CAD build for the part. Positions are in the model's coordinates, mm. Round coordinates to 2 decimals unless told otherwise and drop trailing zeros. Order: outer loops, then holes, each group sorted by start corner. A loop starts at its lowest first (then second) coordinate and runs counter-clockwise, first axis right, second up. Notation, with made-up numbers: (41.5, -16.75) -> (74.5, -16.75) arc R24 ccw to (74.5, -0.75) -> close; hole circle Ø2 at (41, 67). An arc over 180 degrees is marked (long way). Answer as CSV lines item,"result". Start each with the question number.
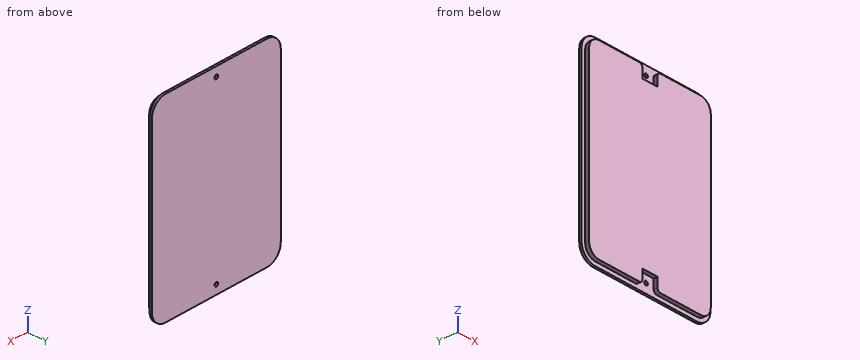
Autodesk Inventor part; units mm, degrees
ref_plane "YZ Plane" through (0, 0, 0) normal (1, 0, 0) x (0, 1, 0)
ref_plane "XZ Plane" through (0, 0, 0) normal (0, 1, 0) x (-1, 0, 0)
ref_plane "XY Plane" through (0, 0, 0) normal (0, 0, 1) x (1, 0, 0)
sketch "Sketch1" plane through (0, 0, 0) normal (0, 1, 0) x (-1, 0, 0)
  line L0 (0, 0) -> (178, 0)
  line L1 (178, 0) -> (178, -248)
  line L2 (178, -248) -> (0, -248)
  line L3 (0, -248) -> (0, 0)
  dimension "d0" = 178
  dimension "d1" = 248
extrude "Extrusion1" add sketch "Sketch1" along normal blind 3
fillet "Fillet1" radius 19 4 edges at (0, 1.5, 0) (-178, 1.5, 0) (0, 1.5, -248) (-178, 1.5, -248)
sketch "Sketch2" plane through (0, 0, 0) normal (0, -1, 0) x (1, 0, 0)
  arc A0 (-178, -229) -> (-159, -248) centre (-159, -229) ccw
  line L0 (-19, -248) -> (-159, -248)
  arc A1 (-19, -248) -> (0, -229) centre (-19, -229) ccw
  line L1 (0, -19) -> (0, -229)
  arc A2 (0, -19) -> (-19, 0) centre (-19, -19) ccw
  line L2 (-159, 0) -> (-19, 0)
  arc A3 (-159, 0) -> (-178, -19) centre (-159, -19) ccw
  line L3 (-178, -229) -> (-178, -19)
  arc A4 (-159, -5) -> (-173, -19) centre (-159, -19) ccw
  line L4 (-159, -5) -> (-19, -5)
  arc A5 (-5, -19) -> (-19, -5) centre (-19, -19) ccw
  line L5 (-5, -19) -> (-5, -229)
  arc A6 (-19, -243) -> (-5, -229) centre (-19, -229) ccw
  line L6 (-19, -243) -> (-159, -243)
  arc A7 (-173, -229) -> (-159, -243) centre (-159, -229) ccw
  line L7 (-173, -229) -> (-173, -19)
  line L8 (-78.5, -243) -> (-99.5, -243)
  line L9 (-99.5, -243) -> (-99.5, -227)
  line L10 (-99.5, -227) -> (-78.5, -227)
  line L11 (-78.5, -227) -> (-78.5, -243)
  line L12 (-173, -124) -> (-5, -124) construction
  line L13 (-78.5, -5) -> (-99.5, -5)
  line L14 (-99.5, -5) -> (-99.5, -21)
  line L15 (-99.5, -21) -> (-78.5, -21)
  line L16 (-78.5, -21) -> (-78.5, -5)
  circle A8 centre (-89, -11.5) radius 2.5
  line L17 (-89, -227) -> (-89, -21) construction
  circle A9 centre (-89, -236.5) radius 2.5
  point P0 (0, 0)
  point P1 (-89, -243)
  point P2 (-89, -5)
  point P3 (-99.5, -243)
  point P4 (-78.5, -5)
  point P5 (-99.5, -5)
  dimension "d12" = 21
  dimension "d13" = 21
  dimension "d14" = 5
  dimension "d16" = 5
  dimension "d18" = 225
extrude "Extrusion2" add sketch "Sketch2" along normal blind 5 contours L4 L14 L15 L16 A5 L5 A6 L6 L11 L10 L9 A7 L7 A4
extrude "Extrusion4" cut sketch "Sketch2" against normal up to surface (3 mm away) contours A8 | A9
fillet "Fillet2" radius 4 4 edges at (-99.5, -2.5, -243) (-78.5, -2.5, -243) (-99.5, -2.5, -5) (-78.5, -2.5, -5)
equation "\"d5\" = d16"
equation "\"d19\" = d16"
properties part number "case5_3DPrint"
Item 1: Band-saw the part on D-D, the plane z = -236.5. Give the cut face in (x, y).
Item 2: Band-saw the part on B-B, the plane y = -3.5. Give the cut face in (x, z).
Item 3: Pin check, flat tips, straight feed: pin 1 (1.5 mm diameter, centred on y = -1.5, z = -17, fed in from -X); pin 2 (4 mm diameter, centred on x = -54.5, y = -3, fed in from +Z); pin 3 (4 mm diameter, centred on y = -3, z = -235, fed in from -X). Stop position of each tip, or through.
Item 4: Probe line 1 (Z direction, x = -89, y = 1.8); line 2 (Z direction, x = -79, y = -2.25); line 3 (X direction, y = -0.25, z = -194). List the from-to ranges inside material, lowest first.
Item 5: Band-saw the part on A-A, the plane x = -89. Give the cut face in (y, z).
Item 6: Band-saw the part on C-C, the plane x = -61. Give the cut face in (y, z).
Values:
1,outline,"(-176.46, 0) -> (-170.82, 0) -> (-170.82, -5) -> (-99.5, -5) -> (-99.5, 0) -> (-91.5, 0) -> (-91.5, 3) -> (-176.46, 3) -> close; (-86.5, 0) -> (-78.5, 0) -> (-78.5, -5) -> (-7.18, -5) -> (-7.18, 0) -> (-1.54, 0) -> (-1.54, 3) -> (-86.5, 3) -> close"
2,outline,"(-173, -229) arc R14 ccw to (-159, -243) -> (-103.5, -243) arc R4 ccw to (-99.5, -239) -> (-99.5, -227) -> (-78.5, -227) -> (-78.5, -239) arc R4 ccw to (-74.5, -243) -> (-19, -243) arc R14 ccw to (-5, -229) -> (-5, -19) arc R14 ccw to (-19, -5) -> (-74.5, -5) arc R4 ccw to (-78.5, -9) -> (-78.5, -21) -> (-99.5, -21) -> (-99.5, -9) arc R4 ccw to (-103.5, -5) -> (-159, -5) arc R14 ccw to (-173, -19) -> close"
3,pin 1,"x = -172.94"
3,pin 2,"z = -5"
3,pin 3,"x = -172.42"
4,line 1,"-248 to -239, -234 to -14, -9 to 0"
4,line 2,"-227 to -21"
4,line 3,"-173 to -5"
5,outline,"(-5, -227) -> (0, -227) -> (0, -234) -> (3, -234) -> (3, -14) -> (0, -14) -> (0, -21) -> (-5, -21) -> close; (0, -248) -> (3, -248) -> (3, -239) -> (0, -239) -> close; (0, -9) -> (3, -9) -> (3, 0) -> (0, 0) -> close"
6,outline,"(-5, -243) -> (0, -243) -> (0, -248) -> (3, -248) -> (3, 0) -> (0, 0) -> (0, -5) -> (-5, -5) -> close"
